Work out the finished part from the listing and answer in its coordinate system (mm). A direction names the side the tool comes from. Round coordinates to 2 decimals unless told otherwise and drop trailing zeros. Order: outer loops, then holes, each group sorted by start corner. A loop starts at its lowest first (then second) coordinate and runs counter-clockwise, first axis right, second up. Notation, with made-up numbers: (-33, 60) -> (-23, 60) arc R27 ccw to (-23, 78) -> close; hole circle Ø6 at (-40, 26). An arc over 180 degrees is marked (long way). Use a Markdown table: item, result. Add a question column.
Item 1: A cutting plane is placed at C-C, the plane z = -0.25. Determine the outline of the cut face in (x, y), plus the area to 3 significant figures.
Item 2: Find the intervals of material crossed by L1, parallel to Y at x = 0, z = 5.75; L2, parallel to Z at x = 6.25, y = -1.75; L3, parallel to Y at x = 1, z = 6.25, in increasing order. Write a range as [from, to].
Item 3: Flat-ended cylindrical pins translate along their axes: P1, Ø3, axis at x = -2.5, z = 3.5, coming from the -Y side; P2, Ø5, axis at y = 3.5, z = -1, coming from the +X side; P3, Ø2, axis at x = -1.5, y = 0.5, coming from the +Z side. Find the tip coordinate at first contact, or state that the pin passes through.
Item 4: For a pull along X with two mould halves and no side action, classify faces 3 (the flat face through (0, 0, 2)), 4 (the cylindrical face through (7.493, 0.33, -1.479)), 5 (the flat face through (-1.4, 4.5, 7)) as +X half, -X half, draft (parallel to the pull), parting line (faces both ways), or undercut.
Item 5: A cutting plane is placed at D-D, the plane z = 5.25. Determine the outline of the cut face in (x, y), plus the area to 3 significant figures.
Item 6: A cutting plane is placed at A-A, the plane x = 0. Determine the outline of the cut face in (y, z).
Item 7: A tool of negligible diameter and unlimited length cuts with its end or side. For faces 1 (the flat face through (0, 0, -3)), 2 (the cylindrical face through (-0.59, 4.46, 4.54)), from which of +Z, -Z, +X, -X, +Y, -Y can it reach the whole face along a straight path? Write none if from no direction.
from build123d import *

# Parameters (mm, degrees)
SCHIZZO1_R                   = 6
ESTRUSIONE_ESTRUSIONE1_DEPTH = 7
SCHIZZO2_R                   = 4.5
TAGLIO_ESTRUSIONE1_DEPTH     = 5
SCHIZZO3_R                   = 7.5
ESTRUSIONE_ESTRUSIONE2_DEPTH = 3


with BuildPart() as part:
    # Schizzo1 → Estrusione-Estrusione1 (new body)
    with BuildSketch(Plane.XY):
        Circle(SCHIZZO1_R)
    extrude(amount=ESTRUSIONE_ESTRUSIONE1_DEPTH)

    # Schizzo2 → Taglio-Estrusione1 (cut)
    with BuildSketch(Plane.XY.offset(7)):
        Circle(SCHIZZO2_R)
    extrude(amount=-TAGLIO_ESTRUSIONE1_DEPTH, mode=Mode.SUBTRACT)

    # Schizzo3 → Estrusione-Estrusione2 (add)
    with BuildSketch(Plane(origin=(0, 0, 0), x_dir=(-1, 0, 0), z_dir=(0, 0, -1))):
        Circle(SCHIZZO3_R)
    extrude(amount=ESTRUSIONE_ESTRUSIONE2_DEPTH)


solid = part.part
Reported:
| question | item | result |
|---|---|---|
| 1 | outline | circle Ø15 at (0, 0) |
| 1 | area | 177 mm² |
| 2 | L1 | [-6, -4.5], [4.5, 6] |
| 2 | L2 | [-3, 0] |
| 2 | L3 | [-5.92, -4.39], [4.39, 5.92] |
| 3 | P1 | y = -5.92 |
| 3 | P2 | x = 7.43 |
| 3 | P3 | z = 2 |
| 4 | face 3 | undercut |
| 4 | face 4 | parting line |
| 4 | face 5 | draft |
| 5 | outline | circle Ø12 at (0, 0); hole circle Ø9 at (0, 0) |
| 5 | area | 49.5 mm² |
| 6 | outline | (-7.5, -3) -> (7.5, -3) -> (7.5, 0) -> (6, 0) -> (6, 7) -> (4.5, 7) -> (4.5, 2) -> (-4.5, 2) -> (-4.5, 7) -> (-6, 7) -> (-6, 0) -> (-7.5, 0) -> close |
| 7 | face 1 | -Z, +X, -X, +Y, -Y |
| 7 | face 2 | +Z |
